Model file for the job. Use its own axes, mm. A direction names the side the tool comes from. Coordinates: 2 decimals unless noted, no trailing zeros. Write each loop counter-clockwise with the first axis right and the second up, starting at its lowest first coordinate (ties: lowest second). Pieces come first, ordered by that corner, then holes.
Q1. Which spindle directions (+Z, -Z, +X, -X, +Y, -Y) get a long thin tool onto all of the face, cutting with end or side? Do faces 4 (the cylindrical face through (1.034, -75.743, 3.986)), 5 (the flat face through (67, 0, 5)). Say none if no direction does.
Q2. Band-saw the part on B-B, the plane z = 1.95. Write the cut outline in (x, y).
Q3. Drill centre lines: probe 1 along Y at (x, z) = (-2, 3.35) (3 decimals); probe 2 along X at (y, z) = (22, 3.85); probe 3 along Y at (x, z) = (-0.5, 0.5). Where is each one in solid material? Low to high.
Q4. Band-saw the part on C-C, the plane y = -12.5. Write the cut outline in (x, z).
Q5. Band-saw the part on A-A, the plane x = 0. Write the cut outline in (y, z).
Q6. Band-saw the part on D-D, the plane y = 69. Write the cut outline in (x, z).
Q7. Pull direction Y, two halves, no side cores. Call faces 1 (the cylindrical face through (-1.15, 75.74, 3.99)), 2 (the cylindrical face through (-1.25, -79.99, 2.46)), 3 (the flat face through (-69.87, 1, 2)): released by +Y, released by -Y, zero draft, split by the parting line, or undercut.
from build123d import *

# Parameters (mm, degrees)
F1_DEPTH = 5
F2_DEPTH = 3


with BuildPart() as f1:
    # F0 (on Top) → F1 (new body)
    with BuildSketch(Plane.XY):
        with BuildLine():
            Line((64.8992869691, 39.065906503), (69.8129998574, 39.065906503))
            ThreePointArc((69.8129998574, 39.065906503), (-0.0588261188, 79.9999783718), (-69.8703767369, 38.9631935889))
            Line((-69.8703767369, 38.9631935889), (-64.9588376934, 38.9668051747))
            ThreePointArc((-64.9588376934, 38.9668051747), (-0.0578086543, 75.7499779416), (64.8992869691, 39.065906503))
        make_face()
        with BuildLine():
            ThreePointArc((-64.9588376934, 38.9668051747), (-67.5890599234, 34.2020683392), (-69.8703767369, 29.2607750179))
            Line((-69.8703767369, 29.2607750179), (-69.8703767369, -29.2607750179))
            ThreePointArc((-69.8703767369, -29.2607750179), (-67.5890599234, -34.2020683392), (-64.9588376934, -38.9668051747))
            Line((-64.9588376934, -38.9668051747), (-64.8703767369, -38.9668702224))
            Line((-64.8703767369, -38.9668702224), (-64.8703767369, -4.1029528413))
            ThreePointArc((-64.8703767369, -4.1029528413), (-65, 0), (-64.8703767369, 4.1029528413))
            Line((-64.8703767369, 4.1029528413), (-64.8703767369, 38.9668702224))
            Line((-64.8703767369, 38.9668702224), (-64.9588376934, 38.9668051747))
        make_face()
        with BuildLine():
            Line((-64.9588376934, 38.9668051747), (-69.8703767369, 38.9631935889))
            Line((-69.8703767369, 38.9631935889), (-69.8703767369, 29.2607750179))
            ThreePointArc((-69.8703767369, 29.2607750179), (-67.5890599234, 34.2020683392), (-64.9588376934, 38.9668051747))
        make_face()
        with BuildLine():
            Line((-69.8703767369, -29.2607750179), (-69.8703767369, -38.9631935889))
            Line((-69.8703767369, -38.9631935889), (-64.9588376934, -38.9668051747))
            ThreePointArc((-64.9588376934, -38.9668051747), (-67.5890599234, -34.2020683392), (-69.8703767369, -29.2607750179))
        make_face()
        with BuildLine():
            ThreePointArc((-69.8703767369, -38.9631935889), (-0.0588261188, -79.9999783718), (69.8129998574, -39.065906503))
            Line((69.8129998574, -39.065906503), (64.8992869691, -39.065906503))
            ThreePointArc((64.8992869691, -39.065906503), (-0.0578086543, -75.7499779416), (-64.9588376934, -38.9668051747))
            Line((-64.9588376934, -38.9668051747), (-69.8703767369, -38.9631935889))
        make_face()
        with BuildLine():
            Line((69.8129998574, -29.397407214), (69.8129998574, 29.397407214))
            ThreePointArc((69.8129998574, 29.397407214), (67.5294011904, 34.3197097142), (64.8992869691, 39.065906503))
            Line((64.8992869691, 39.065906503), (64.8992869691, 3.6169809102))
            ThreePointArc((64.8992869691, 3.6169809102), (64.9748168639, 1.8091913953), (65, 0))
            ThreePointArc((65, 0), (64.9748168639, -1.8091913953), (64.8992869691, -3.6169809102))
            Line((64.8992869691, -3.6169809102), (64.8992869691, -39.065906503))
            ThreePointArc((64.8992869691, -39.065906503), (67.5294011904, -34.3197097142), (69.8129998574, -29.397407214))
        make_face()
        with BuildLine():
            Line((64.8992869691, -39.065906503), (69.8129998574, -39.065906503))
            Line((69.8129998574, -39.065906503), (69.8129998574, -29.397407214))
            ThreePointArc((69.8129998574, -29.397407214), (67.5294011904, -34.3197097142), (64.8992869691, -39.065906503))
        make_face()
        with BuildLine():
            Line((69.8129998574, 29.397407214), (69.8129998574, 39.065906503))
            Line((69.8129998574, 39.065906503), (64.8992869691, 39.065906503))
            ThreePointArc((64.8992869691, 39.065906503), (67.5294011904, 34.3197097142), (69.8129998574, 29.397407214))
        make_face()
    extrude(amount=F1_DEPTH)

    # F0 (on Top) → F2 (join)
    with BuildSketch(Plane.XY):
        with BuildLine():
            ThreePointArc((-64.9588376934, -38.9668051747), (-0.0578086543, -75.7499779416), (64.8992869691, -39.065906503))
            Line((64.8992869691, -39.065906503), (64.8992869691, -3.6169809102))
            ThreePointArc((64.8992869691, -3.6169809102), (0.2434155497, -64.9995442205), (-64.8703767369, -4.1029528413))
            Line((-64.8703767369, -4.1029528413), (-64.8703767369, -38.9668702224))
            Line((-64.8703767369, -38.9668702224), (-64.9588376934, -38.9668051747))
        make_face()
        with BuildLine():
            Line((64.8992869691, 3.6169809102), (64.8992869691, 39.065906503))
            ThreePointArc((64.8992869691, 39.065906503), (-0.0578086543, 75.7499779416), (-64.9588376934, 38.9668051747))
            Line((-64.9588376934, 38.9668051747), (-64.8703767369, 38.9668702224))
            Line((-64.8703767369, 38.9668702224), (-64.8703767369, 4.1029528413))
            ThreePointArc((-64.8703767369, 4.1029528413), (0.2434155497, 64.9995442205), (64.8992869691, 3.6169809102))
        make_face()
    extrude(amount=F2_DEPTH)


solid = f1.part
Answer sheet:
1. face 4: +Z
1. face 5: +Z, +X, -X, +Y, -Y
2. outline: (-69.87, -38.96) arc R80 ccw to (69.81, -39.07) - (69.81, 39.07) arc R80 ccw to (-69.87, 38.96) - close; hole circle Ø130 at (0, 0)
3. probe 1: y = -79.975 to -75.724, 75.724 to 79.975
3. probe 2: x = -69.87 to -64.87, 64.9 to 69.81
3. probe 3: y = -80 to -65, 65 to 80
4. outline: (-69.87, 0) - (-63.79, 0) - (-63.79, 3) - (-64.87, 3) - (-64.87, 5) - (-69.87, 5) - close; (63.79, 0) - (69.81, 0) - (69.81, 5) - (64.9, 5) - (64.9, 3) - (63.79, 3) - close
5. outline: (-80, 0) - (-65, 0) - (-65, 3) - (-75.75, 3) - (-75.75, 5) - (-80, 5) - close; (65, 0) - (80, 0) - (80, 5) - (75.75, 5) - (75.75, 3) - (65, 3) - close
6. outline: (-40.48, 0) - (40.48, 0) - (40.48, 5) - (31.26, 5) - (31.26, 3) - (-31.26, 3) - (-31.26, 5) - (-40.48, 5) - close
7. face 1: undercut
7. face 2: released by -Y
7. face 3: zero draft
